Build history of the part. All positions in model axes, mm. A direction names the side the tool comes from. Round coordinates to 2 decimals unless told otherwise and drop trailing zeros. Loops run counter-clockwise (first coordinate to the right, second up) from the corner with the lowest first, then second, coordinate; pieces in that order, holes last.
from build123d import *

# Parameters (mm, degrees)
TORUS_R           = 2
CYLINDER001_R     = 2.1
CYLINDER001_DEPTH = 10
ARRAY_X_COUNT     = 2
ARRAY_X_PITCH     = 77
ARRAY_Y_COUNT     = 2
ARRAY_Y_PITCH     = 62
PAD002_DEPTH      = 3
CYLINDER_R        = 7
CYLINDER_DEPTH    = 20


with BuildPart() as torus:
    # Torus → Torus (revolve)
    with BuildSketch(Plane(origin=(0, 0, 15), x_dir=(1, 0, 0), z_dir=(0, -1, 0))):
        with Locations((7, 0)):
            Circle(TORUS_R)
    revolve(axis=Axis((0, 0, 15), (0, 0, 1)))


with BuildPart() as extract_fusion:
    # Cylinder001 → Cylinder001 (new body)
    with BuildSketch(Plane.XY):
        Circle(CYLINDER001_R)
    extrude(amount=CYLINDER001_DEPTH)

    # Array X: extract fusion ×2


with BuildPart() as extract_fusion_1:
    add(extract_fusion.part)
    with Locations(*[(i * ARRAY_X_PITCH, 0, 0) for i in range(1, ARRAY_X_COUNT)]):
        add(extract_fusion.part)

    # Array Y: extract fusion ×2


with BuildPart() as extract_fusion_2:
    add(extract_fusion_1.part)
    with Locations(*[(0, i * ARRAY_Y_PITCH, 0) for i in range(1, ARRAY_Y_COUNT)]):
        add(extract_fusion_1.part)


with BuildPart() as extract_fusion_3:
    # Array placement: moved
    add(extract_fusion_2.part.moved(Location((-38.5, -31, 0))))

    # Fusion: union Torus
    add(torus.part)


with BuildPart() as base_body:
    # Sketch002 → Pad002 (new body)
    with BuildSketch(Plane.XY):
        with BuildLine():
            Line((-10.285127, -3.90079), (-41.474221, -26.980795))
            ThreePointArc((-41.474221, -26.980795), (-42.519205, -33.974221), (-35.525779, -35.019205))
            Line((-35.525779, -35.019205), (-3.650353, -11.431313))
            ThreePointArc((-3.650353, -11.431313), (0, -12), (3.650353, -11.431313))
            Line((3.650353, -11.431313), (35.525779, -35.019205))
            ThreePointArc((35.525779, -35.019205), (42.519205, -33.974221), (41.474221, -26.980795))
            Line((10.285127, -3.90079), (41.474221, -26.980795))
            ThreePointArc((10.285127, -3.90079), (11, 0), (10.285127, 3.90079))
            Line((10.285127, 3.90079), (41.474221, 26.980795))
            ThreePointArc((41.474221, 26.980795), (42.519205, 33.974221), (35.525779, 35.019205))
            Line((3.650353, 11.431313), (35.525779, 35.019205))
            ThreePointArc((3.650353, 11.431313), (0, 12), (-3.650353, 11.431313))
            Line((-3.650353, 11.431313), (-35.525779, 35.019205))
            ThreePointArc((-35.525779, 35.019205), (-42.519205, 33.974221), (-41.474221, 26.980795))
            Line((-10.285127, 3.90079), (-41.474221, 26.980795))
            ThreePointArc((-10.285127, 3.90079), (-11, 0), (-10.285127, -3.90079))
        make_face()
    extrude(amount=PAD002_DEPTH)


with BuildPart() as base_cut:
    # Cylinder → Cylinder (new body)
    with BuildSketch(Plane.XY):
        Circle(CYLINDER_R)
    extrude(amount=CYLINDER_DEPTH)

    # Fusion001: union base body
    add(base_body.part)

    # Cut: cut extract fusion
    add(extract_fusion_3.part, mode=Mode.SUBTRACT)


solid = base_cut.part
(1) Pull direction Y, two halves, no side cores. Call faces 4 (the face through (-42.58, -33.89, 1.48)), 5 (the face through (-7, -5, 3)), 6 (the face through (6.466, -2.681, 7.93)), 7 (the face through (19.365, -23.06, 1.479)): +Y half, -Y half, draft (parallel to the pull), parting line (faces both ways), or undercut.
Responses:
face 4: undercut
face 5: draft
face 6: parting line
face 7: -Y half
(2) Pin check, flat tips, straight feed: P1, Ø8, axis at x = 10, y = 25.5, coming from the +Z side; P2, Ø4, axis at x = 2, z = 17.5, coming from the +Y side; P3, Ø10, axis at x = -16, y = 2.5, coming from the +Z side; P4, Ø1.5, axis at y = 1.5, z = 5.5, coming from the -X side. Stop position of each tip, or through.
Responses:
P1: passes through
P2: stops at y = 7
P3: stops at z = 3
P4: stops at x = -6.96
(3) Slice it at A-A on y = -31. List the corners of the cut face in (x, z), plus the area to 3 significant figures.
Responses:
outline: (-43.5, 0) - (-40.6, 0) - (-40.6, 3) - (-43.5, 3) - close; (-36.4, 0) - (-30.09, 0) - (-30.09, 3) - (-36.4, 3) - close; (30.09, 0) - (36.4, 0) - (36.4, 3) - (30.09, 3) - close; (40.6, 0) - (43.5, 0) - (43.5, 3) - (40.6, 3) - close
area: 55.2 mm2
(4) Slice it at B-B on z = 1.5. List the corners of the cut face in (x, y).
Responses:
outline: (-41.47, -26.98) arc R5 ccw to (-35.53, -35.02) - (-3.65, -11.43) arc R12 ccw to (3.65, -11.43) - (35.53, -35.02) arc R5 ccw to (41.47, -26.98) - (10.29, -3.9) arc R11 ccw to (10.29, 3.9) - (41.47, 26.98) arc R5 ccw to (35.53, 35.02) - (3.65, 11.43) arc R12 ccw to (-3.65, 11.43) - (-35.53, 35.02) arc R5 ccw to (-41.47, 26.98) - (-10.29, 3.9) arc R11 ccw to (-10.29, -3.9) - close; hole circle Ø4.2 at (-38.5, -31); hole circle Ø4.2 at (-38.5, 31); hole circle Ø4.2 at (38.5, -31); hole circle Ø4.2 at (38.5, 31)
(5) Which spindle directions (+Z, -Z, +X, -X, +Y, -Y) get a long thin tool onto all of the face, cutting with end or side? Do faces 1 (the face through (19.365, 23.06, 1.479)), 2 (the face through (-25.66, -15.28, 1.48)), 3 (the face through (6.466, -2.681, 18.479)). Say none if no direction does.
Responses:
face 1: +Z, -Z, +Y
face 2: +Z, -Z, -X
face 3: +Z
(6) Slice it at C-C on x = 0. List the corners of the cut face in (y, z), plus the area to 3 significant figures.
Responses:
outline: (-12, 0) - (12, 0) - (12, 3) - (7, 3) - (7, 13) arc R2 cw to (7, 17) - (7, 20) - (-7, 20) - (-7, 17) arc R2 cw to (-7, 13) - (-7, 3) - (-12, 3) - close
area: 297 mm2
(7) Slice it at D-D on x = -38.5. List the corners of the cut face in (y, z).
Responses:
outline: (-36, 0) - (-33.1, 0) - (-33.1, 3) - (-36, 3) - close; (-28.9, 0) - (-24.78, 0) - (-24.78, 3) - (-28.9, 3) - close; (24.78, 0) - (28.9, 0) - (28.9, 3) - (24.78, 3) - close; (33.1, 0) - (36, 0) - (36, 3) - (33.1, 3) - close
(8) Probe line 1 (X direction, y = 31, z = 1.85); line 2 (Y direction, x = -38.5, z = 1.85); line 3 (Z direction, x = 19, y = 17). List the from-to ranges inside material, lowest first.
Responses:
line 1: x = -43.5 to -40.6, -36.4 to -30.09, 30.09 to 36.4, 40.6 to 43.5
line 2: y = -36 to -33.1, -28.9 to -24.78, 24.78 to 28.9, 33.1 to 36
line 3: z = 0 to 3
